from build123d import *

# Parameters (mm, degrees)
SKETCH2_OUTSIDE_W  = 53.474
SKETCH2_OUTSIDE_H  = 53.474
CUT_EXTRUDE1_DEPTH = 3
SKETCH3_OUTSIDE_W  = 53.474
SKETCH3_OUTSIDE_H  = 53.474
CUT_EXTRUDE2_DEPTH = 4
SKETCH4_OUTSIDE_W  = 50.37
SKETCH4_OUTSIDE_H  = 50.37
CUT_EXTRUDE3_DEPTH = 8


with BuildPart() as part:
    # Sketch1 → Revolve1 (revolve)
    with BuildSketch(Plane.XY, mode=Mode.PRIVATE) as revolve1_sk:
        Polygon((30, 0), (-109, 0), (-109, 2), (-107, 2), (-107, 3.5), (-105.5, 6.098076211), (-104, 3.5), (-104, 2), (-102, 2), (-102, 3.5), (-100.5, 6.098076211), (-99, 3.5), (-99, 2), (-94, 2), (-94, 10), (0, 10), (0, 6), (7, 6), (7, 8), (9, 11.464101615), (11, 8), (11, 6), (12, 6), (12, 5), (20, 5), (20, 2), (23, 2), (23, 3.5), (24.5, 6.098076211), (26, 3.5), (26, 2), (30, 2), align=None)
    revolve(revolve1_sk.sketch.rotate(Axis((30, 0, 0), (1, 0, 0)), 90), axis=Axis((30, 0, 0), (1, 0, 0)))

    # Sketch2 outside → Cut-Extrude1 (cut)
    with BuildSketch(Plane(origin=(26, 0, 0), x_dir=(0, 0, -1), z_dir=(1, 0, 0))):
        Rectangle(SKETCH2_OUTSIDE_W, SKETCH2_OUTSIDE_H)
        Polygon((0, -4.618802154), (4, -2.309401077), (4, 2.309401077), (0, 4.618802154), (-4, 2.309401077), (-4, -2.309401077), align=None, mode=Mode.SUBTRACT)
    extrude(amount=-CUT_EXTRUDE1_DEPTH, mode=Mode.SUBTRACT)

    # Sketch3 outside → Cut-Extrude2 (cut)
    with BuildSketch(Plane(origin=(11, 0, 0), x_dir=(0, 0, -1), z_dir=(1, 0, 0))):
        Rectangle(SKETCH3_OUTSIDE_W, SKETCH3_OUTSIDE_H)
        Polygon((0, 9.814954576), (-8.5, 4.907477288), (-8.5, -4.907477288), (0, -9.814954576), (8.5, -4.907477288), (8.5, 4.907477288), align=None, mode=Mode.SUBTRACT)
    extrude(amount=-CUT_EXTRUDE2_DEPTH, mode=Mode.SUBTRACT)

    # Sketch4 outside → Cut-Extrude3 (cut)
    with BuildSketch(Plane.ZY.offset(107)):
        Rectangle(SKETCH4_OUTSIDE_W, SKETCH4_OUTSIDE_H)
        Polygon((0, 4.618802154), (-4, 2.309401077), (-4, -2.309401077), (0, -4.618802154), (4, -2.309401077), (4, 2.309401077), align=None, mode=Mode.SUBTRACT)
    extrude(amount=-CUT_EXTRUDE3_DEPTH, mode=Mode.SUBTRACT)


solid = part.part
Geometry check sheet. Reference: the model listing, model coordinates, mm. A direction names the side the tool comes from. Coordinates: 2 decimals unless noted, no trailing zeros. Order: outer loops, then holes, each group sorted by start corner. A loop starts at its lowest first (then second) coordinate and runs counter-clockwise, first axis right, second up. Notation, with made-up numbers: (78.25, 26) - (119.25, 26) arc R10 ccw to (119.25, 34) - close; hole circle Ø9 at (48.5, 9). An arc over 180 degrees is marked (long way). Answer in a Markdown table with one row per item. Add a question column.
1) Gauge pin test, flat ends, axial feed: P1, Ø1.2, axis at x = -100.5, y = 0, coming from the -Z side; P2, Ø5.5, axis at y = -1.5, z = -1.5, coming from the -X side; P3, Ø4, axis at x = 14.5, z = 4, coming from the -Y side; P4, Ø3, axis at x = -82, z = -3, coming from the +Y side. Record the tip position at first contact, or that the pin passes through.
2) Cross-section at A-A, the plane x = -16. Record the cut outline in (y, z).
3) Set-up check for faces 1 (the cylindrical face through (28, 2, 0)), 2 (the flat face through (-101, 0, -4)), 3 (the flat face through (24.52, -3.48, -1.97)), 4 (the flat face through (-105.52, -3.48, 1.97)): record each of +Z, -Z, +X, -X, +Y, -Y from which the full face is reachable in a straight line by a thin tool's end or side.
4) Material ranges on line 1 along X through (y, z) = (-0.75, 2.75); line 2 along X through (y, z) = (4.75, -7); line 3 along X through (y, z) = (-3.25, -6.5), recorded low to high. Write a range as [from, to].
Check result:
| question | item | result |
|---|---|---|
| 1 | P1 | stops at z = -4 |
| 1 | P2 | stops at x = -109 |
| 1 | P3 | stops at y = -4.58 |
| 1 | P4 | stops at y = 9.89 |
| 2 | outline | circle Ø20 at (0, 0) |
| 3 | face 1 | +X |
| 3 | face 2 | -Z, -X, +Y, -Y |
| 3 | face 3 | -Z, +X, -Y |
| 3 | face 4 | +Z, -X, -Y |
| 4 | line 1 | x = [-107, -104], [-102, -99], [-94, 20], [23, 26] |
| 4 | line 2 | x = [-94, 0], [7.27, 10.73] |
| 4 | line 3 | x = [-94, 0], [7, 11] |
